Source: three-view drawing plus pictorial views. Frame: mm from the lowest corner of the part. A direction names the side the tool comes from. Round coordinates to 2 decimals unless told otherwise and drop trailing zeros. Loops run counter-clockwise (first coordinate to the right, second up) from the corner with the lowest first, then second, coordinate; pieces in that order, holes last. Notation, with made-up numbers: (-15, 57.5) -> (-7, 57.5) arc R19 ccw to (-7, 92.5) -> close; hole circle Ø1 at (-18.75, 84.5). An arc over 180 degrees is marked (long way). Answer as a JSON object with one key per item and string values. Group by question number.
Item 1: Draft query along X for the marked faces 1, 2 and 3. Return one class per face: released by +X, released by -X, zero draft, split by the parting line, or undercut.
Item 2: Pin query (flat end, axial travel): pin 1 (8 mm diameter, centred on y = 757.5, z = 570, fed in from -X); pin 2 (12 mm diameter, centred on x = 368, y = 467.5, fed in from -Z); pin 3 (1 mm diameter, centred on x = 1196, y = 1312, fed in from +Z); pin 4 (1 mm diameter, centred on x = 522, z = 632.5, fed in from -Y). Return the tip coordinate at first contact, or that it passes through.
Item 3: Section query C-C on z = 514. Return loops of the section in (x, y), and give its area (3 significant figures).
Item 4: Section query A-A on x = 762. Return loops of the section in (y, z).
Item 5: Set-up query: the marked faces 4 and 5. Return all of +Z, -Z, +X, -X, +Y, -Y with unobstructed straight access to the full face (end or side cutting, diameter ignored); none if empty.
Item 6: Material intervals for line 1 (Y direction, x = 762, z = 106); line 2 (Z direction, x = 1240, y = 378); line 3 (X direction, y = 645, z = 618), sorted ascending. Write a range as [from, to].
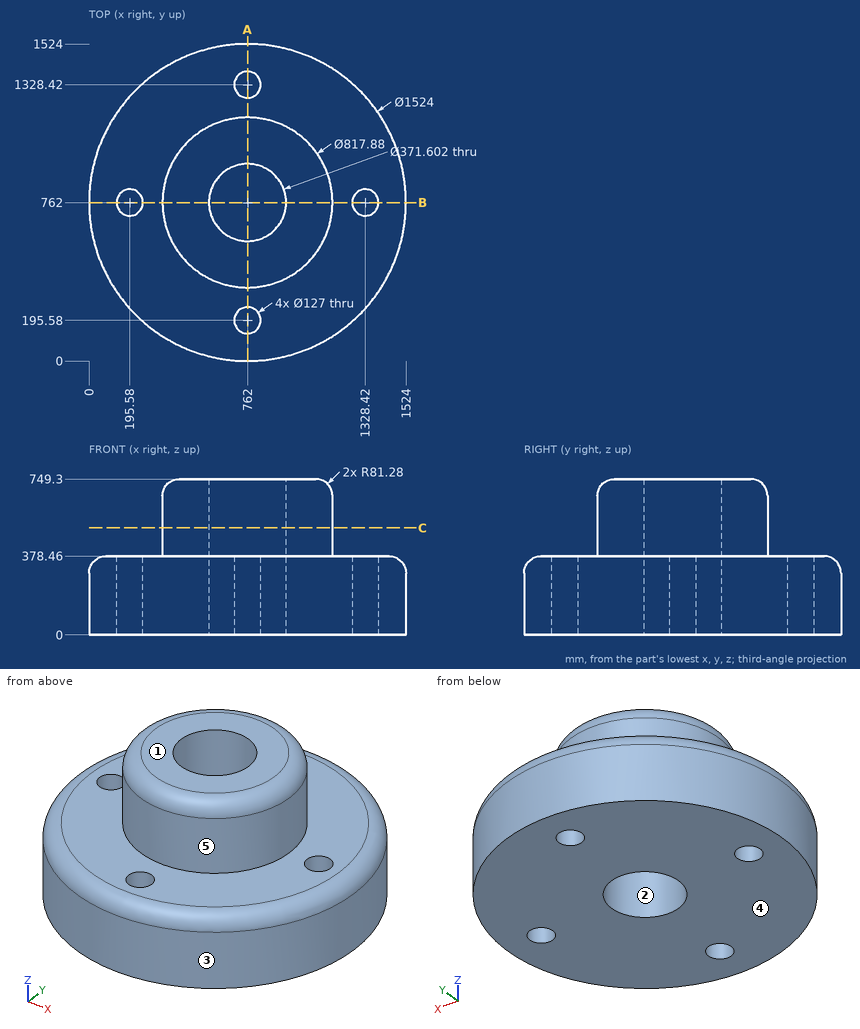
Solved:
{
 "1": {"face 1": "zero draft", "face 2": "undercut", "face 3": "split by the parting line"},
 "2": {"pin 1": "x = 353.06", "pin 2": "z = 0", "pin 3": "z = 376.11", "pin 4": "y = 430.53"},
 "3": {"outline": "circle Ø817.88 at (762, 762); hole circle Ø371.6 at (762, 762)", "area": "417,000 mm²"},
 "4": {"outline": "(0, 0) -> (132.08, 0) -> (132.08, 378.46) -> (81.28, 378.46) arc R81.28 ccw to (0, 297.18) -> close; (259.08, 0) -> (576.2, 0) -> (576.2, 749.3) -> (434.34, 749.3) arc R81.28 ccw to (353.06, 668.02) -> (353.06, 378.46) -> (259.08, 378.46) -> close; (947.8, 0) -> (1264.92, 0) -> (1264.92, 378.46) -> (1170.94, 378.46) -> (1170.94, 668.02) arc R81.28 ccw to (1089.66, 749.3) -> (947.8, 749.3) -> close; (1391.92, 0) -> (1524, 0) -> (1524, 297.18) arc R81.28 ccw to (1442.72, 378.46) -> (1391.92, 378.46) -> close"},
 "5": {"face 4": "-Z, +X, -X, +Y, -Y", "face 5": "+Z"},
 "6": {"line 1": "[0, 132.08], [259.08, 576.2], [947.8, 1264.92], [1391.92, 1524]", "line 2": "[0, 378.46]", "line 3": "[370.15, 617.66], [906.34, 1153.85]"}
}
